from build123d import *

# Parameters (mm, degrees)
F1_START = 12.7
F1_DEPTH = 88.9
F3_DEPTH = 0.8001


# Not quite as in the source:
# - a feature names something its author has since deleted; it is built from what else it names


with BuildPart() as f1:
    # F0 (on Front) → F1 (new body)
    with BuildSketch(Plane.XZ.offset(F1_START)):
        with BuildLine():
            ThreePointArc((-1.5875, 1.5875), (-1.1225320151, 0.4649679849), (0, 0))
            Line((0, 0), (15.8496, 0))
            ThreePointArc((15.8496, 0), (16.9721320151, 0.4649679849), (17.4371, 1.5875))
            Line((17.4371, 1.5875), (16.637, 1.5875))
            ThreePointArc((16.637, 1.5875), (16.4063758795, 1.0307241205), (15.8496, 0.8001))
            Line((15.8496, 0.8001), (7.9248, 0.8001))
            Line((7.9248, 0.8001), (0, 0.8001))
            ThreePointArc((0, 0.8001), (-0.5567758795, 1.0307241205), (-0.7874, 1.5875))
            Line((-0.7874, 1.5875), (-1.5875, 1.5875))
        make_face()
    extrude(amount=F1_DEPTH)

    # F2 (on face) → F3 (cut, through all)
    with BuildSketch(Plane.XY.offset(0.8001)):
        with BuildLine():
            Line((4.7498, -33.8666666667), (7.9248, -33.8666666667))
            Line((7.9248, -33.8666666667), (6.8115473336, -30.8932353995))
            ThreePointArc((6.8115473336, -30.8932353995), (5.3156619991, -32.0575166198), (4.7498, -33.8666666667))
        make_face()
        with BuildLine():
            Line((7.9248, -33.8666666667), (11.0998, -33.8666666667))
            ThreePointArc((11.0998, -33.8666666667), (9.7339500469, -31.2575286657), (6.8115473336, -30.8932353995))
            Line((6.8115473336, -30.8932353995), (7.9248, -33.8666666667))
        make_face()
        with BuildLine():
            ThreePointArc((4.7498, -33.8666666667), (7.9248, -37.0416666667), (11.0998, -33.8666666667))
            Line((11.0998, -33.8666666667), (7.9248, -33.8666666667))
            Line((7.9248, -33.8666666667), (4.7498, -33.8666666667))
        make_face()
    extrude(amount=-F3_DEPTH, mode=Mode.SUBTRACT)


solid = f1.part
The model under review builds one solid part; all positions refer to its coordinate system, in mm. Round coordinates to 2 decimals unless told otherwise and drop trailing zeros. Order: outer loops, then holes, each group sorted by start corner. A loop starts at its lowest first (then second) coordinate and runs counter-clockwise, first axis right, second up. Notation, with made-up numbers: (84, 89.25) -> (112, 89.25) arc R25 cw to (112, 106.25) -> close; hole circle Ø4 at (7, 30.25). An arc over 180 degrees is marked (long way). Use CSV: the item, a comma, the result in double quotes. Start each with the question number.
(1) Consider section C-C on x = 13.5. Write out the cut boundary in (y, z).
(2) Consider section B-B on z = 1.15. Write out the cut boundary in (x, y).
(3) Consider section A-A on y = -94. Write out the cut boundary in (x, z) (1 decimal), and give its area (3 significant figures).
(4) Wall thickness on probe 1 along Z at (x, y) = (5, -72); probe 2 along X at (y, z) = (-79, 1.1); probe 3 along X at (y, z) = (-64, 0.95): over which ranges is each line inside the solid? List them lowest first. Write a range as from..to.
(5) Mouldability with a two-part tool opening along X and no side actions: class faces 1 (the face through (8, -57, 0.8)), 2 (the face through (-1.135, -56.528, 0.477)), 3 (the face through (8, -57, 0)) as pulls with the +X half, pulls with the -X half, needs draft (parallel to the pull), parting line crosses it, or undercut.
(6) Insertion check: pin 1 (1 mm diameter, centred on x = 13, y = -74.5, fed in from +Z). The pin has a flat end and moves straight along its axis. Give the tip position at first contact, or say it passes through.
Responses:
1,outline,"(-101.6, 0) -> (-12.7, 0) -> (-12.7, 0.8) -> (-101.6, 0.8) -> close"
2,outline,"(-1.53, -101.6) -> (-0.65, -101.6) -> (-0.65, -12.7) -> (-1.53, -12.7) -> close; (16.5, -101.6) -> (17.38, -101.6) -> (17.38, -12.7) -> (16.5, -12.7) -> close"
3,outline,"(-1.6, 1.6) arc R1.6 ccw to (0, 0) -> (15.8, 0) arc R1.6 ccw to (17.4, 1.6) -> (16.6, 1.6) arc R0.8 cw to (15.8, 0.8) -> (0, 0.8) arc R0.8 cw to (-0.8, 1.6) -> close"
3,area,"15.7 mm²"
4,probe 1,"0..0.8"
4,probe 2,"-1.51..-0.62, 16.47..17.36"
4,probe 3,"-1.45..-0.46, 16.31..17.3"
5,face 1,"undercut"
5,face 2,"pulls with the -X half"
5,face 3,"needs draft"
6,pin 1,"z = 0.8"
